from build123d import *

# Parameters (mm, degrees)
F0_R     = 37
F0_R_2   = 20
F0_R_3   = 2.65
F0_R_4   = 4
F1_DEPTH = 8
F2_DEPTH = 2


# Not quite as in the source:
# - a feature names something its author has since deleted; it is built from what else it names


with BuildPart() as f1:
    # F0 (on Right) → F1 (new body)
    with BuildSketch(Plane.YZ):
        Circle(F0_R)
        Circle(F0_R_2, mode=Mode.SUBTRACT)
        Circle(F0_R_2)
        with Locations((-12.5573683549, -7.25)):
            Circle(F0_R_3, mode=Mode.SUBTRACT)
        with Locations((12.5573683549, -7.25)):
            Circle(F0_R_3, mode=Mode.SUBTRACT)
        Circle(F0_R_4, mode=Mode.SUBTRACT)
        with Locations((0, 14.5)):
            Circle(F0_R_3, mode=Mode.SUBTRACT)
    extrude(amount=-F1_DEPTH)

    # F0 (on Right) → F2 (cut)
    with BuildSketch(Plane.YZ):
        Circle(F0_R)
        Circle(F0_R_2, mode=Mode.SUBTRACT)
    extrude(amount=-F2_DEPTH, mode=Mode.SUBTRACT)


solid = f1.part
The listing builds one solid part. Answer for the finished solid, in the listing's coordinates (mm). A direction names the side the tool comes from. Coordinates: 2 decimals unless noted, no trailing zeros. Loops run counter-clockwise (first coordinate to the right, second up) from the corner with the lowest first, then second, coordinate; pieces in that order, holes last. Notation, with made-up numbers: (82.5, 81.25) -> (141.5, 81.25) arc R20 cw to (141.5, 109.25) -> close; hole circle Ø11 at (66, 23). An arc over 180 degrees is marked (long way). Write item = value, one per line. Start each with the question number.
1) A tool of negligible diameter and unlimited length cuts with its end or side. For faces 1 (the face through (-2, 16, -16)), 2 (the face through (0, 4.2, 0.3)), from which of +Z, -Z, +X, -X, +Y, -Y can it reach the whole face along a straight path? Write none if from no direction.
2) The mould has two halves that part along Z. Classify faces 3 (the face through (-4.96, -8.02, -36.12)), 4 (the face through (-8, -1, -8)), 5 (the face through (-3.944, 11.983, -9.837)): released by +Z, released by -Z, zero draft, split by the parting line, or undercut.
3) Given pin 1 Ø1.5 at (x, z) = (-4.5, 6) entering from +Y; pin 2 Ø2 at (x, y) = (-6, 10) entering from +Z; pin 3 Ø3 at (x, z) = (-6, 2.5) entering from -Y; pin 4 Ø6 at (y, z) = (0, 14.5) entering from +X, each flat-ended and moving along its own axis, determine where each tip first touches the part or whether it passes through.
4) A cutting plane is placed at A-A (z = 0). Give the vertices of the cut face in (x, y).
5) A cutting plane is placed at B-B (y = 0). Give the vertices of the cut face in (x, z).
6) A cutting plane is placed at C-C (x = -6). Give the vertices of the cut face in (y, z), then the cut area to 3 significant figures.
7) A cutting plane is placed at D-D (z = -18). Give the vertices of the cut face in (x, y), then the cut area to 3 significant figures.
8) Straight lines are drawn through the part: line 1 (Z direction, x = -2.25, y = 0); line 2 (Y direction, x = -2.5, z = -8.5); line 3 (Y direction, x = -6.25, z = -5.5). For each, find the intervals that lie inside material, in ascending order. Write a range as from..to.
Responses:
q1.face_1 = +X
q1.face_2 = +Z, -Z, +X, +Y, -Y
q2.face_3 = split by the parting line
q2.face_4 = zero draft
q2.face_5 = undercut
q3.pin_1 = 36.63
q3.pin_2 = 35.89
q3.pin_3 = -36.99
q3.pin_4 = 0
q4.outline = (-8, -37) -> (-2, -37) -> (-2, -20) -> (0, -20) -> (0, -4) -> (-8, -4) -> close; (-8, 4) -> (0, 4) -> (0, 20) -> (-2, 20) -> (-2, 37) -> (-8, 37) -> close
q5.outline = (-8, -37) -> (-2, -37) -> (-2, -20) -> (0, -20) -> (0, -4) -> (-8, -4) -> close; (-8, 4) -> (0, 4) -> (0, 11.85) -> (-8, 11.85) -> close; (-8, 17.15) -> (0, 17.15) -> (0, 20) -> (-2, 20) -> (-2, 37) -> (-8, 37) -> close
q6.outline = circle Ø74 at (0, 0); hole circle Ø5.3 at (-12.56, -7.25); hole circle Ø8 at (0, 0); hole circle Ø5.3 at (0, 14.5); hole circle Ø5.3 at (12.56, -7.25)
q6.area = 4,180 mm²
q7.outline = (-8, -32.33) -> (-2, -32.33) -> (-2, -8.72) -> (0, -8.72) -> (0, 8.72) -> (-2, 8.72) -> (-2, 32.33) -> (-8, 32.33) -> close
q7.area = 423 mm²
q8.line_1 = -37..-4, 4..11.85, 17.15..37
q8.line_2 = -36.01..-14.89, -10.22..10.22, 14.89..36.01
q8.line_3 = -36.59..-14.55, -10.57..10.57, 14.55..36.59
